For this review, use the dimensioned drawing (mm, ordinates from the lowest corner) and the shaded views. A direction names the side the tool comes from. Coordinates: 2 decimals unless noted, no trailing zeros. Loops run counter-clockwise (first coordinate to the right, second up) from the corner with the lowest first, then second, coordinate; pieces in that order, holes last. Notation, with made-up numbers: (-16, 13) - (-9, 13) arc R21 ccw to (-9, 31) - close; hole circle Ø5 at (68.5, 83). An arc over 180 degrees is marked (long way). One line per item, written item: value. Start each with the question number.
1. We need section D-D, the plane y = 7. Give the boundary of the cut face in (x, z) (1 decimal).
2. For the marked faces 1, 2 and 3, list the 3-axis set-ups (+Z, -Z, +X, -X, +Y, -Y) from which the entire face can be reached by the end or side of a thin tool; tool diameter is ignored.
3. We need section C-C, the plane y = 3.5. Give the boundary of the cut face in (x, z), then the cut area to 3 significant figures.
4. Insertion check: P1, Ø0.8, axis at x = 2, z = 1, coming from the +Y side; P2, Ø1.4, axis at x = 1.5, y = 3, coming from the +Z side; P3, Ø1.5, axis at x = 7.5, z = 1, coming from the +Y side. Each pin has a flat end and moves straight along its axis. Give the tip position at first contact, or say it passes through.
5. To check wall thickness, follow line 1 (Y direction, x = 4.8, z = 1.85); line 2 (X direction, y = 4.75, z = 0.45); line 3 (Y direction, x = 4.8, z = 0.95). State the ranges of each line that lie inside material, in increasing order.
6. We need section B-B, the plane x = 4. Give the boundary of the cut face in (y, z).
7. Mouldability with a two-part tool opening along X and no side actions: class the marked faces 4, 5, 6 and 7 as +X half, -X half, draft (parallel to the pull), parting line (faces both ways), or undercut.
8. We need section A-A, the plane z = 1. Give the boundary of the cut face in (x, y) (1 decimal).
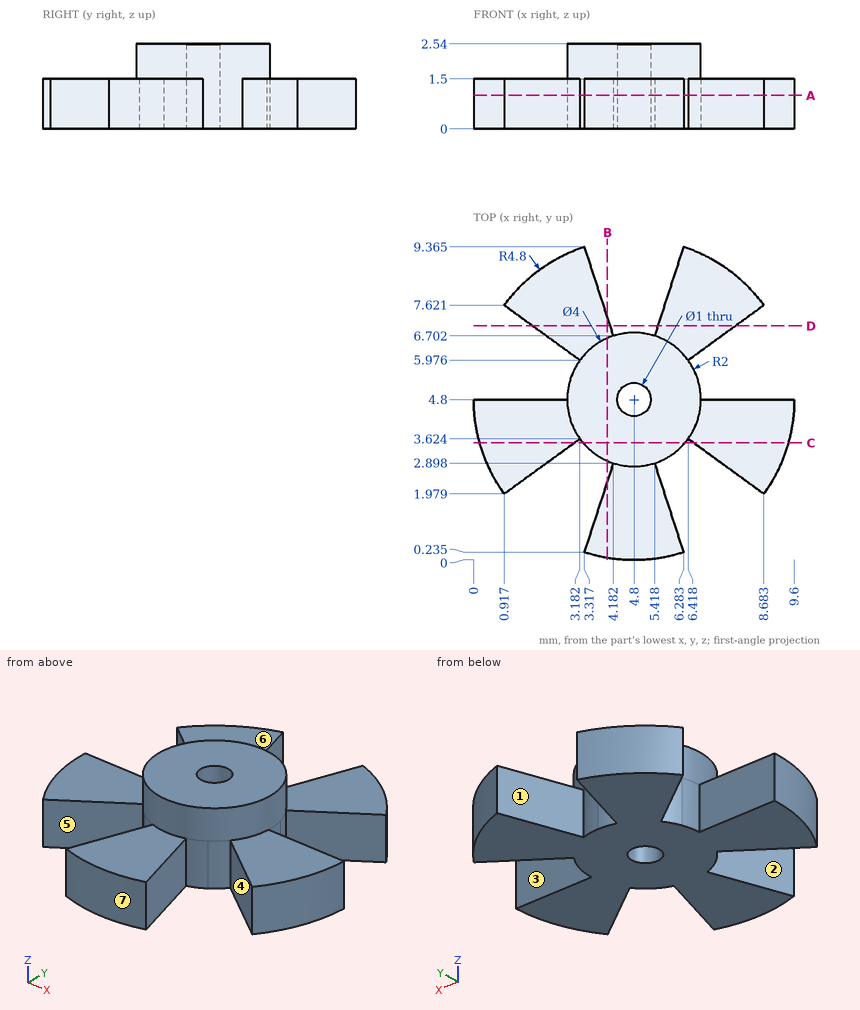
Findings below:
1. outline: (1.8, 0) - (4.1, 0) - (4.1, 1.5) - (1.8, 1.5) - close; (5.5, 0) - (7.8, 0) - (7.8, 1.5) - (5.5, 1.5) - close
2. face 1: +Z, -Z, +Y
2. face 2: +Z, -Z
2. face 3: +Z, -Z, +X
3. outline: (0.18, 0) - (3.01, 0) - (3.01, 1.5) - (0.18, 1.5) - close; (3.28, 0) - (6.32, 0) - (6.32, 2.54) - (3.28, 2.54) - close; (6.59, 0) - (9.42, 0) - (9.42, 1.5) - (6.59, 1.5) - close
3. area: 16.2 mm2
4. P1: y = 8.96
4. P2: z = 1.5
4. P3: y = 9.19
5. line 1: 2.8 to 4.3, 5.3 to 6.8
5. line 2: 0 to 4.3, 5.3 to 9.6
5. line 3: 0 to 4.3, 5.3 to 6.8
6. outline: (0.07, 0) - (2.34, 0) - (2.34, 1.5) - (0.07, 1.5) - close; (2.97, 0) - (7.26, 0) - (7.26, 1.5) - (6.63, 1.5) - (6.63, 2.54) - (2.97, 2.54) - close
7. face 4: undercut
7. face 5: undercut
7. face 6: draft
7. face 7: parting line
8. outline: (0, 4.8) arc R4.8 ccw to (0.9, 2) - (3.2, 3.6) arc R2 ccw to (4.2, 2.9) - (3.3, 0.2) arc R4.8 ccw to (6.3, 0.2) - (5.4, 2.9) arc R2 ccw to (6.4, 3.6) - (8.7, 2) arc R4.8 ccw to (9.6, 4.8) - (6.8, 4.8) arc R2 ccw to (6.4, 6) - (8.7, 7.6) arc R4.8 ccw to (6.3, 9.4) - (5.4, 6.7) arc R2 ccw to (4.2, 6.7) - (3.3, 9.4) arc R4.8 ccw to (0.9, 7.6) - (3.2, 6) arc R2 ccw to (2.8, 4.8) - close; hole circle Ø1 at (4.8, 4.8)
